Geometry check sheet. Reference: drawing and pictorial views, mm from the part's lowest x, y, z. A direction names the side the tool comes from. Give positions to 0.01 mm unless a question says otherwise; leave off trailing zeros. Write each loop counter-clockwise with the first axis right and the second up, starting at its lowest first coordinate (ties: lowest second). Pieces come first, ordered by that corner, then holes. Notation, with made-up numbers: (-33.5, 85) -> (-28.5, 85) arc R23 cw to (-28.5, 119) -> close; hole circle Ø4 at (72.25, 48). An arc over 180 degrees is marked (long way). Return JSON: item names as keys, results as strings.
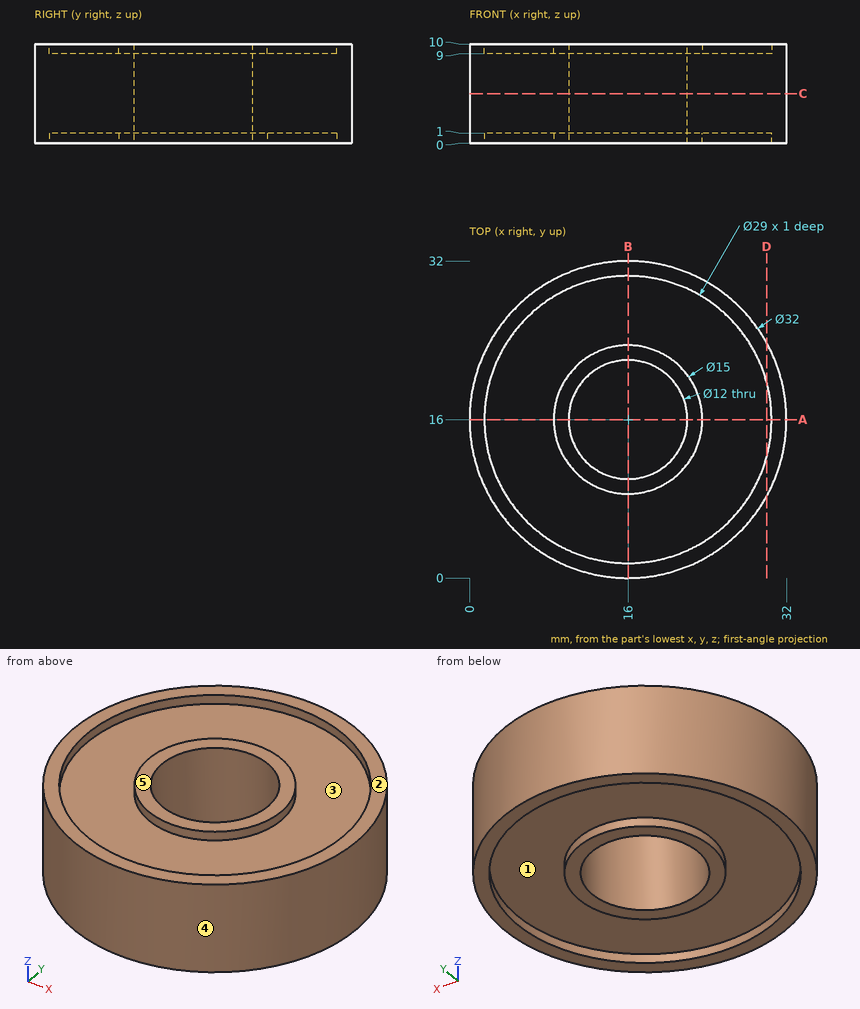
(1) Thickness scan on L1, parallel to Y at x = 16, z = 9.75; L2, parallel to Y at x = 16, z = 6; L3, parallel to Z at x = 19.5, y = 29. Record the ranges inside material, lowest first.
Reply:
{"L1": "0 to 1.5, 8.5 to 10, 22 to 23.5, 30.5 to 32", "L2": "0 to 10, 22 to 32", "L3": "1 to 9"}
(2) Cross-section at D-D on x = 30. Enter the section's corners in (y, z), then the cut area to 3 significant figures.
Reply:
{"outline": "(8.25, 0) -> (12.23, 0) -> (12.23, 1) -> (19.77, 1) -> (19.77, 0) -> (23.75, 0) -> (23.75, 10) -> (19.77, 10) -> (19.77, 9) -> (12.23, 9) -> (12.23, 10) -> (8.25, 10) -> close", "area": "140 mm^2"}
(3) Release check for a two-part mould opening along X. For the marked faces 3, 4 and 5 record: pulls with the +X half, pulls with the -X half, needs draft (parallel to the pull), parting line crosses it, or undercut.
Reply:
{"face 3": "undercut", "face 4": "parting line crosses it", "face 5": "needs draft"}
(4) Depth check by flat-ended pin: pin 1 Ø3 at (x, y) = (11, 7) entering from -Z; pin 2 Ø2 at (x, z) = (11, 4) entering from -Y; pin 3 Ø1 at (y, z) = (22, 7.5) entering from -X (3 decimals). Enter the tip coordinate at first touch or a pass-through.
Reply:
{"pin 1": "z = 1", "pin 2": "y = 0.51", "pin 3": "x = 0.975"}
(5) Set-up check for the marked faces 1 and 2: record each of +Z, -Z, +X, -X, +Y, -Y from which the full face is reachable in a straight line by a thin tool's end or side.
Reply:
{"face 1": "-Z", "face 2": "+Z, +X, -X, +Y, -Y"}
(6) Cross-section at A-A on y = 16. Enter the section's corners in (x, z), then the cut area to 3 significant figures.
Reply:
{"outline": "(0, 0) -> (1.5, 0) -> (1.5, 1) -> (8.5, 1) -> (8.5, 0) -> (10, 0) -> (10, 10) -> (8.5, 10) -> (8.5, 9) -> (1.5, 9) -> (1.5, 10) -> (0, 10) -> close; (22, 0) -> (23.5, 0) -> (23.5, 1) -> (30.5, 1) -> (30.5, 0) -> (32, 0) -> (32, 10) -> (30.5, 10) -> (30.5, 9) -> (23.5, 9) -> (23.5, 10) -> (22, 10) -> close", "area": "172 mm^2"}
(7) Cross-section at C-C on z = 5. Enter the section's corners in (x, y).
Reply:
{"outline": "circle Ø32 at (16, 16); hole circle Ø12 at (16, 16)"}
